Design review of the part built by this model. Coordinates are the model's own, in mm. Give positions to 0.01 mm unless a question says otherwise; leave off trailing zeros. Write each loop counter-clockwise with the first axis right and the second up, starting at its lowest first coordinate (ties: lowest second). Pieces come first, ordered by that corner, then holes. Notation, with made-up numbers: (49, 14) -> (108, 14) arc R25 ccw to (108, 32) -> close; hole circle Ø1 at (30, 55). An arc over 180 degrees is marked (long way). Answer as a JSON object with one key per item and string values.
Autodesk Inventor part; units mm, degrees
ref_plane "Plano de trabajo3" through (41.55, 0, 0) normal (1, 0, 0) x (0, 1, 0)
ref_plane "XZ Plane" through (0, 0, 0) normal (0, 1, 0) x (-1, 0, 0)
ref_plane "XY Plane" through (0, 0, 0) normal (0, 0, 1) x (1, 0, 0)
sketch "Boceto1" plane through (0, 0, 0) normal (1, 0, 0) x (0, 1, 0)
  circle A0 centre (0, 0) radius 7.85
  dimension "d0" = 15.7
ref_plane "Plano de trabajo1" through (11.225, 0, 0) normal (1, 0, 0) x (0, 1, 0)
sketch "Boceto2" plane through (11.225, 0, 0) normal (1, 0, 0) x (0, 1, 0)
  circle A0 centre (0, 0) radius 19.075
  dimension "d2" = 38.15
ref_plane "Plano de trabajo2" through (30.325, 0, 0) normal (1, 0, 0) x (0, 1, 0)
sketch "Boceto3" plane through (30.325, 0, 0) normal (1, 0, 0) x (0, 1, 0)
  point P0 (0, 0)
ref_plane "Plano de trabajo3" through (41.55, 0, 0) normal (1, 0, 0) x (0, 1, 0)
sketch "Boceto4" plane through (41.55, 0, 0) normal (1, 0, 0) x (0, 1, 0)
  circle A0 centre (0, 0) radius 7.85
  dimension "d6" = 15.7
extrude "Extrusión1" add sketch "Boceto2" along normal blind 19.1
extrude "Extrusión2" add sketch "Boceto1" along normal blind 15
extrude "Extrusión3" add sketch "Boceto4" against normal blind 15
loft "Solevación1" add section 1 edges at (41.55, -7.85, 0) section 2 edges at (30.325, -19.075, 0)
loft "Solevación2" add section 1 edges at (0, -7.85, 0) section 2 edges at (11.225, -19.075, 0)
properties part number "PESAS BAILARINA"
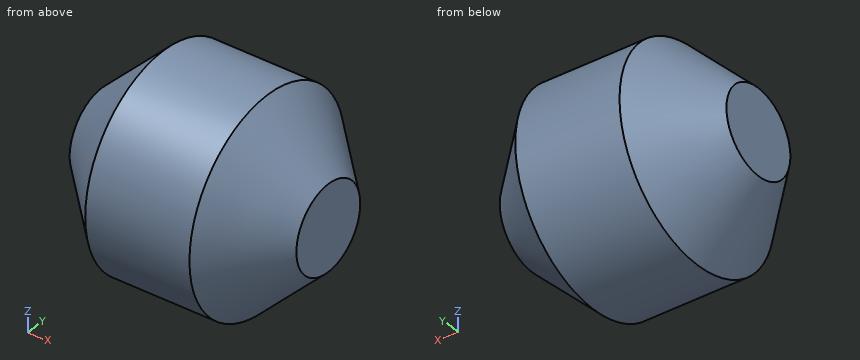
(1) Clearance check with flat-ended pins moving along their axes: pin 1 (1.5 mm diameter, centred on x = 25, z = -2, fed in from -Y); pin 2 (12 mm diameter, centred on x = 16.5, z = -13.5, fed in from +Y); pin 3 (1.5 mm diameter, centred on x = 8, z = 9, fed in from -Y); pin 4 (5 mm diameter, centred on y = -6, z = -7.5, fed in from +X). State where each tip first meets the part, or that it passes through.
Here are the results:
{"pin 1": "stops at y = -19.03", "pin 2": "stops at y = 17.54", "pin 3": "stops at y = -14.07", "pin 4": "stops at x = 41.55"}
(2) We need section C-C, the plane x = 35. State the section outline as (y, z) points, then the cut area to 3 significant figures.
Here are the results:
{"outline": "circle Ø28.8 at (0, 0)", "area": "651 mm²"}
(3) For line 1 along Z through (x, y) = (28.5, 0) (3 decimals); line 2 along Y through (x, z) = (10, -4); line 3 along Z through (x, y) = (18.5, -7.5), list the stretches that pass through material, from the lowest coordinate up.
Here are the results:
{"line 1": "z = -19.075 to 19.075", "line 2": "y = -17.4 to 17.4", "line 3": "z = -17.54 to 17.54"}
(4) We need section A-A, the plane y = 0. State the section outline as (x, z) points (3 decimals), then the cut area to 3 significant figures.
Here are the results:
{"outline": "(0, -7.85) -> (11.225, -19.075) -> (30.325, -19.075) -> (41.55, -7.85) -> (41.55, 7.85) -> (30.325, 19.075) -> (11.225, 19.075) -> (0, 7.85) -> close", "area": "1,330 mm²"}
(5) We need section B-B, the plane x = 6.5. State the section outline as (y, z) points, then the cut area to 3 significant figures.
Here are the results:
{"outline": "circle Ø28.7 at (0, 0)", "area": "647 mm²"}
